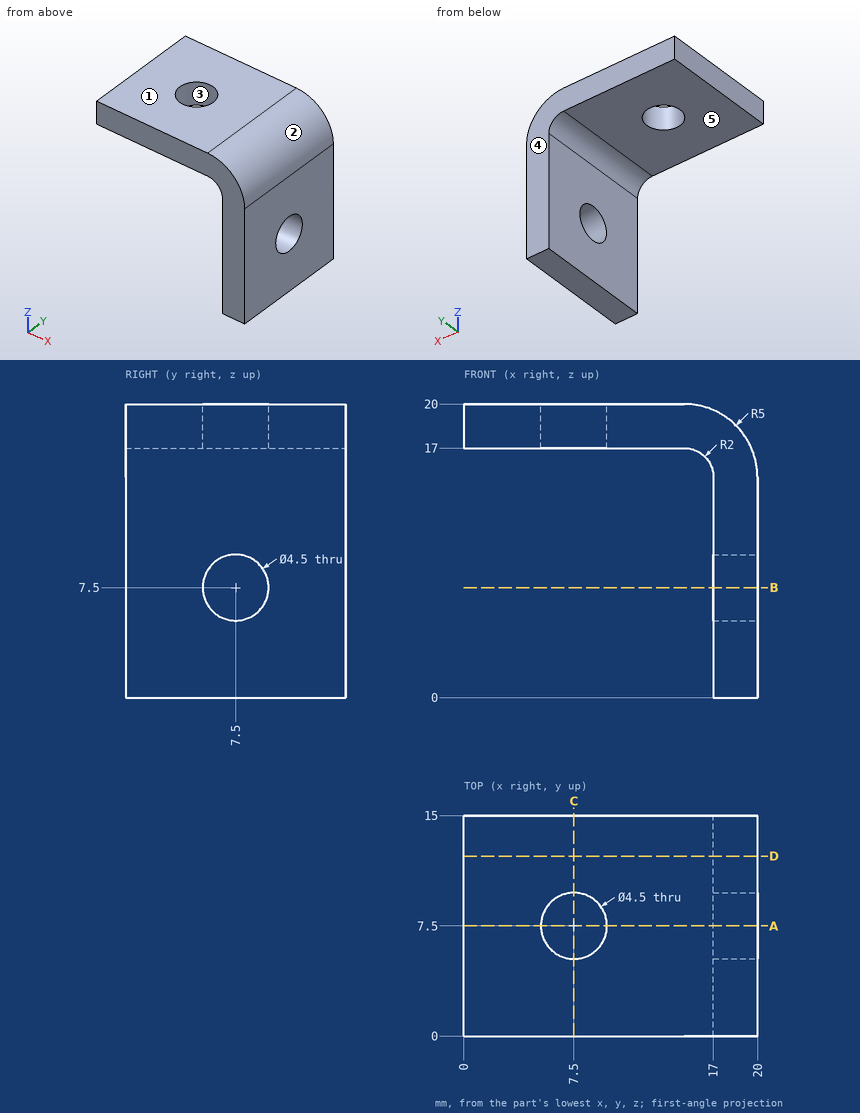
Print and shaded views of the part. All mm, measured from the part's lowest x, y and z. A direction names the side the tool comes from. Round coordinates to 2 decimals unless told otherwise and drop trailing zeros. Write each loop counter-clockwise with the first axis right and the second up, starting at its lowest first coordinate (ties: lowest second). Pieces come first, ordered by that corner, then holes. Notation, with made-up numbers: M 74.25,55.5 L 98.25,55.5 A23 cw 98.25,94.5 Z; hole C 15.5,17.5 d4. An arc over 180 degrees is marked long. Use a Markdown table: item, result. Add a question column.
1. Pull direction X, two halves, no side cores. Call the marked faces 1, 2 and 3: released by +X, released by -X, zero draft, split by the parting line, or undercut.
2. Slice it at C-C on x = 7.5. Give the cut face in (y, z), then the cut area to 3 significant figures.
3. Drill centre lines: probe 1 along Y at (x, z) = (18.9, 7.5); probe 2 along X at (y, z) = (6.5, 9.75). Where is each one in solid material? Low to high.
4. Slice it at A-A on y = 7.5. Give the cut face in (x, z), then the cut area to 3 significant figures.
5. Slice it at B-B on z = 7.5. Give the cut face in (x, y).
6. 3-axis set-ups, long thin cutter, end or side, ignore diameter. For the marked faces 4 and 5: which of +Z, -Z, +X, -X, +Y, -Y reach the whole face in a straight line?
7. Flat gauge pins, fed straight in: P1, Ø3, axis at y = 10, z = 10.5, coming from the -X side; P2, Ø1.5, axis at y = 7, z = 7.5, coming from the -X side; P3, Ø1, axis at x = 17, y = 5.5, coming from the +Z side; P4, Ø4, axis at x = 9.5, y = 9.5, coming from the -Z side. Where does each tip first touch, or does it go through?
8. Slice it at D-D on y = 12.25. Give the cut face in (x, z).
Reply:
| question | item | result |
|---|---|---|
| 1 | face 1 | zero draft |
| 1 | face 2 | released by +X |
| 1 | face 3 | undercut |
| 2 | outline | M 0,17 L 5.25,17 L 5.25,20 L 0,20 Z; M 9.75,17 L 15,17 L 15,20 L 9.75,20 Z |
| 2 | area | 31.5 mm^2 |
| 3 | probe 1 | y = 0 to 5.25, 9.75 to 15 |
| 3 | probe 2 | x = 17 to 20 |
| 4 | outline | M 0,17 L 5.25,17 L 5.25,20 L 0,20 Z; M 9.75,17 L 15,17 A2 cw 17,15 L 17,9.75 L 20,9.75 L 20,15 A5 ccw 15,20 L 9.75,20 Z; M 17,0 L 20,0 L 20,5.25 L 17,5.25 Z |
| 4 | area | 79.5 mm^2 |
| 5 | outline | M 17,0 L 20,0 L 20,5.25 L 17,5.25 Z; M 17,9.75 L 20,9.75 L 20,15 L 17,15 Z |
| 6 | face 4 | +Z, -Z, +X, -X, +Y |
| 6 | face 5 | -Z, -X, +Y, -Y |
| 7 | P1 | stops at x = 17 |
| 7 | P2 | passes through |
| 7 | P3 | stops at z = 19.77 |
| 7 | P4 | stops at z = 17 |
| 8 | outline | M 0,17 L 15,17 A2 cw 17,15 L 17,0 L 20,0 L 20,15 A5 ccw 15,20 L 0,20 Z |
